Drawing for the job (mm, zero at the part's lowest x, y, z). A direction names the side the tool comes from. Give positions to 0.01 mm unless a question says otherwise; leave off trailing zeros. Order: outer loops, then holes, each group sorted by start corner. A loop starts at its lowest first (then second) coordinate and runs counter-clockwise, first axis right, second up. Notation, with made-up numbers: (-27, 87.5) -> (-3, 87.5) arc R32 ccw to (-3, 114.5) -> close; hole circle Ø11 at (-37, 59.5). An arc over 180 degrees is marked (long way). Use one line per item in the form item = value. Start each with the question number.
1) Probe line 1 (Z direction, x = 63.5, y = 20.25); line 2 (Z direction, x = 12.7, y = 7); line 3 (X direction, y = 11.25, z = 60) (1 decimal). List the from-to ranges inside material, lowest first.
2) Cut at B-B, the plane x = 88.9. State how many separate pieces and enclosed holes the cut face has, and give its area (3 significant figures).
3) Cut at A-A, the plane z = 31.75. Give the cut face in (x, y).
4) Cut at D-D, the plane x = 38.1. Give the cut face in (y, z).
5) Tool access for the marked faces 1, 2 and 3: list every direction of +Z, -Z, +X, -X, +Y, -Y with a clear straight run to the whole face (end or side of a thin tool).
6) Drop flat-ended pins along their axis: P1, Ø5.5, axis at x = 86, z = 13, coming from the -Y side (1 decimal); P2, Ø1, axis at x = 24, y = 8, coming from the -Z side; P3, Ø3.5, axis at x = 87, z = 58.5, coming from the +Y side; P4, Ø6, axis at x = 38.1, z = 31.75, coming from the +Y side. Give the stop position or say it passes through.
7) Mould opens along X. For the marked faces 4, 5 and 6 say: pulls with the +X half, pulls with the -X half, needs draft (parallel to the pull), parting line crosses it, or undercut.
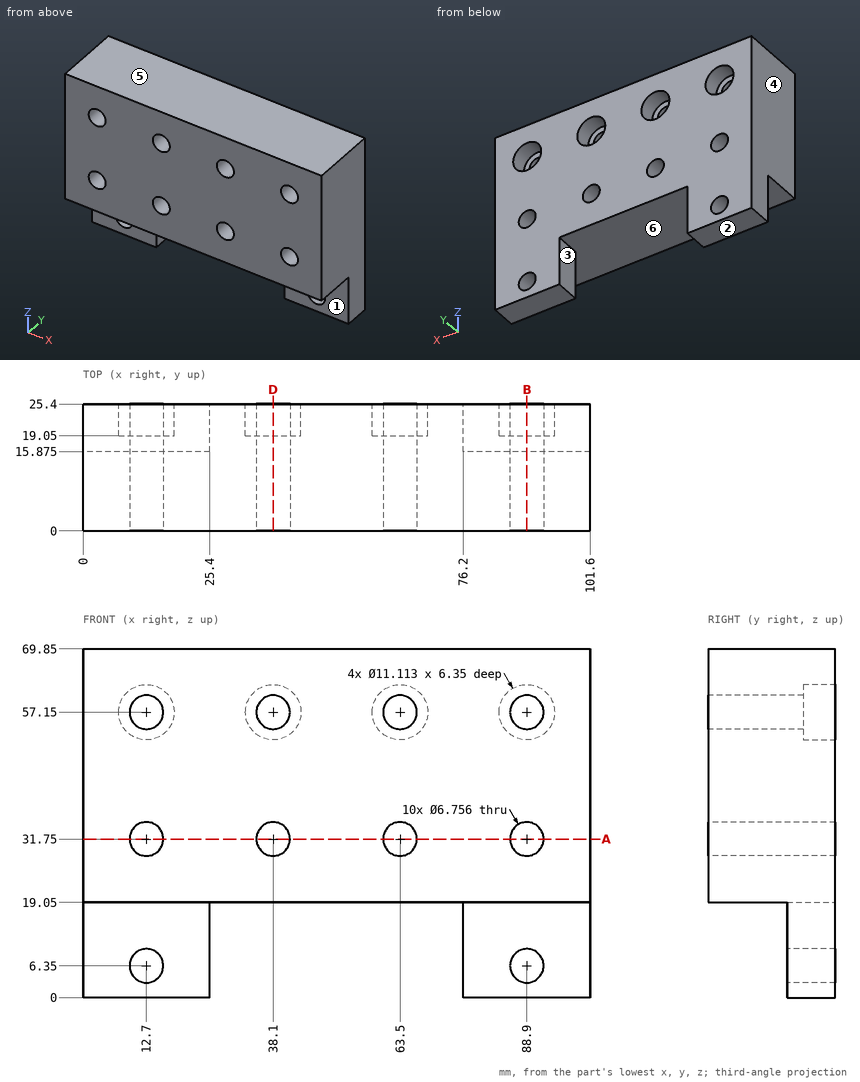
Result:
q1.line_1 = 19.05 to 28.37, 35.13 to 51.59, 62.71 to 69.85
q1.line_2 = 19.05 to 28.37, 35.13 to 53.77, 60.53 to 69.85
q1.line_3 = 0 to 10.9, 14.5 to 36.3, 39.9 to 61.7, 65.3 to 87.1, 90.7 to 101.6
q2.separate_pieces = 4
q2.enclosed_holes = 0
q2.area = 1,040 mm²
q3.outline = (0, 0) -> (9.32, 0) -> (9.32, 25.4) -> (0, 25.4) -> close; (16.08, 0) -> (34.72, 0) -> (34.72, 25.4) -> (16.08, 25.4) -> close; (41.48, 0) -> (60.12, 0) -> (60.12, 25.4) -> (41.48, 25.4) -> close; (66.88, 0) -> (85.52, 0) -> (85.52, 25.4) -> (66.88, 25.4) -> close; (92.28, 0) -> (101.6, 0) -> (101.6, 25.4) -> (92.28, 25.4) -> close
q4.outline = (0, 19.05) -> (25.4, 19.05) -> (25.4, 28.37) -> (0, 28.37) -> close; (0, 35.13) -> (25.4, 35.13) -> (25.4, 51.59) -> (19.05, 51.59) -> (19.05, 53.77) -> (0, 53.77) -> close; (0, 60.53) -> (19.05, 60.53) -> (19.05, 62.71) -> (25.4, 62.71) -> (25.4, 69.85) -> (0, 69.85) -> close
q5.face_1 = -Z, +X, -X, -Y
q5.face_2 = -Z, +X, -X, +Y, -Y
q5.face_3 = -Z, +Y, -Y
q6.P1 = 15.9
q6.P2 = 19.05
q6.P3 = 19.05
q6.P4 = through
q7.face_4 = pulls with the -X half
q7.face_5 = needs draft
q7.face_6 = undercut
